Design review of the part built by this model. Coordinates are the model's own, in mm. Face numbers are marked on the shaded views. Give positions to 0.01 mm unless a question says otherwise; leave off trailing zeros. Loops run counter-clockwise (first coordinate to the right, second up) from the corner with the lowest first, then second, coordinate; pieces in that order, holes last. Notation, with made-up numbers: (37, 73.25) - (65, 73.25) arc R23 ccw to (65, 103.25) - close; hole circle Ø6 at (81, 87). An arc over 180 degrees is marked (long way). Write each question's results on one line, items separated by ' | '.
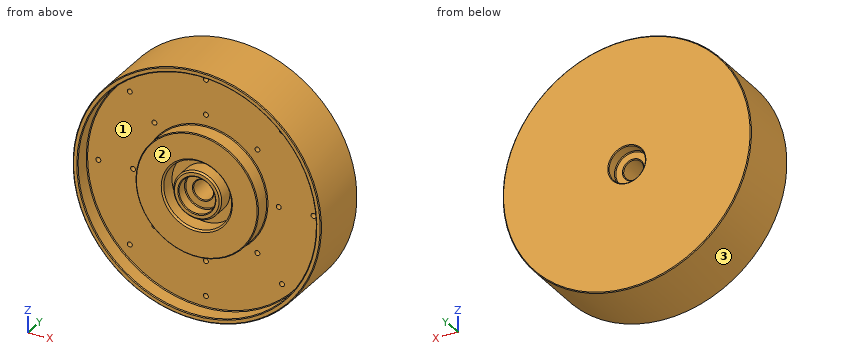
from build123d import *

# Parameters (mm, degrees)
SKETCH3_R          = 1.5
CUT_EXTRUDE1_DEPTH = 15
SKETCH4_R          = 20.5
SKETCH4_R_2        = 14.5
CUT_EXTRUDE2_DEPTH = 10
CHAMFER1_SIZE      = 1


with BuildPart() as part:
    # Sketch2 → Revolve1 (revolve)
    with BuildSketch(Plane(origin=(0, 0, 0), x_dir=(0, 0, -1), z_dir=(1, 0, 0))):
        Polygon((-6, 12.5), (-6, -12.5), (-6.5, -13), (-10.5, -13), (-11, -13.5), (-11, -19.5), (-11.5, -20), (-36.5, -20), (-37, -19.5), (-37, -10.5), (-37.5, -10), (-71.5, -10), (-72, -10.5), (-72, -19.5), (-72.5, -20), (-74.5, -20), (-75, -19.5), (-75, 19.5), (-74.5, 20), (-72.5, 20), (-37, 20), (-36.5, 20), (-11.5, 20), (-11, 19.5), (-11, 13.5), (-10.5, 13), (-6.5, 13), align=None)
    revolve(axis=Axis((0, 77.621858512, 0), (0, -1, 0)))

    # Sketch3 → Cut-Extrude1 (cut)
    with BuildSketch(Plane.XZ.offset(10)):
        with Locations(Location((-45.961940777, 45.961940777, 0), (0, 0, 270))):
            Circle(SKETCH3_R)
        with Locations(Location((-31.112698372, 31.112698372, 0), (0, 0, 270))):
            Circle(SKETCH3_R)
        with Locations(Location((31.112698372, 31.112698372, 0), (0, 0, 270))):
            Circle(SKETCH3_R)
        with Locations(Location((45.961940777, 45.961940777, 0), (0, 0, 270))):
            Circle(SKETCH3_R)
        with Locations(Location((-65, 0, 0), (0, 0, 270))):
            Circle(SKETCH3_R)
        with Locations(Location((-44, 0, 0), (0, 0, 270))):
            Circle(SKETCH3_R)
        with Locations(Location((-45.961940777, -45.961940777, 0), (0, 0, 270))):
            Circle(SKETCH3_R)
        with Locations(Location((-31.112698372, -31.112698372, 0), (0, 0, 270))):
            Circle(SKETCH3_R)
        with Locations(Location((0, -44, 0), (0, 0, 270))):
            Circle(SKETCH3_R)
        with Locations(Location((0, -65, 0), (0, 0, 270))):
            Circle(SKETCH3_R)
        with Locations(Location((31.112698372, -31.112698372, 0), (0, 0, 270))):
            Circle(SKETCH3_R)
        with Locations(Location((45.961940777, -45.961940777, 0), (0, 0, 270))):
            Circle(SKETCH3_R)
        with Locations(Location((44, 0, 0), (0, 0, 270))):
            Circle(SKETCH3_R)
        with Locations(Location((65, 0, 0), (0, 0, 270))):
            Circle(SKETCH3_R)
        with Locations(Location((0, 44, 0), (0, 0, 270))):
            Circle(SKETCH3_R)
        with Locations(Location((0, 65, 0), (0, 0, 270))):
            Circle(SKETCH3_R)
    extrude(amount=-CUT_EXTRUDE1_DEPTH, mode=Mode.SUBTRACT)

    # Sketch4 → Cut-Extrude2 (cut)
    with BuildSketch(Plane(origin=(0, -20, 0), x_dir=(1, 0, 0), z_dir=(0, 1, 0))):
        with Locations(Location((0, 0, 0), (0, 0, 270))):
            Circle(SKETCH4_R)
        with Locations(Location((0, 0, 0), (0, 0, 270))):
            Circle(SKETCH4_R_2, mode=Mode.SUBTRACT)
    extrude(amount=CUT_EXTRUDE2_DEPTH, mode=Mode.SUBTRACT)

    # Chamfer1
    chamfer1_edges = [part.edges().sort_by_distance(p)[0] for p in [
        (0, -20, -14.5),
        (0, -20, -20.5),
    ]]
    chamfer(chamfer1_edges, length=CHAMFER1_SIZE)


solid = part.part
(1) Take a section at B-B on y = -4. Count the separate pieces of the cut face and the enclosed holes in it, plus the area to 3 significant figures.
Answers below:
separate pieces: 1 | enclosed holes: 17 | area: 17,400 mm2
(2) Wall thickness on line 1 along X through (y, z) = (-3.75, 0); line 2 along Z through (x, y) = (-46, 2); line 3 along X through (y, z) = (-15, -24): over which ranges is each line inside the solid? List them lowest first. Write a range as from..to.
Answers below:
line 1: -75..-66.5, -63.5..-45.5, -42.5..-6, 6..42.5, 45.5..63.5, 66.5..75 | line 2: -59.24..-47.46, -44.46..44.46, 47.46..59.24 | line 3: -71.06..-67.88, -28.16..28.16, 67.88..71.06
(3) Insertion check: P1, Ø4, axis at y = 5, z = 17, coming from the +X side; P2, Ø2, axis at x = -10, z = -40, coming from the -Y side; P3, Ø23, axis at x = -3.5, z = -1, coming from the +Y side; P4, Ø8, axis at x = -12.5, y = -10, coming from the -Z side. Each pin has a flat end and moves straight along its axis. Give the tip position at first contact, or say it passes through.
Answers below:
P1: x = 73.48 | P2: y = -10 | P3: y = 20 | P4: z = -74.52
(4) Draft analysis for pull direction X (two halves, no side actions). For the marked faces 1, 2 and 3, state which applies: pulls with the +X half, pulls with the -X half, needs draft (parallel to the pull), parting line crosses it, or undercut.
Answers below:
face 1: undercut | face 2: needs draft | face 3: parting line crosses it
(5) Take a section at C-C on y = 7.5. Give the boundary of the cut face in (x, z).
Answers below:
outline: circle Ø150 at (0, 0); hole circle Ø12 at (0, 0)
(6) Take a section at A-A on y = -17. Give the boundary of the cut face in (x, z), plus the area to 3 significant figures.
Answers below:
outline: circle Ø150 at (0, 0); circle Ø74 at (0, 0); circle Ø29 at (0, 0); hole circle Ø144 at (0, 0); hole circle Ø41 at (0, 0); hole circle Ø22 at (0, 0) | area: 4,650 mm2
(7) Take a section at D-D on y = 15.5. Give the boundary of the cut face in (x, z), plus the area to 3 significant figures.
Answers below:
outline: circle Ø150 at (0, 0); hole circle Ø22 at (0, 0) | area: 17,300 mm2
